Read the model definition and answer for the solid it produces. Units are mm, in the model's axes. A direction names the side the tool comes from. Coordinates: 2 decimals unless noted, no trailing zeros. Order: outer loops, then holes, each group sorted by start corner. A loop starts at its lowest first (then second) coordinate and runs counter-clockwise, first axis right, second up. Notation, with made-up numbers: M 65.25,-0.5 L 111.25,-0.5 A22 ccw 111.25,35.5 Z; hole C 58,40.5 d6. An arc over 180 degrees is marked long. Put each result on its own line as item: value.
from build123d import *

# Parameters (mm, degrees)
SKETCH1_R             = 2.25
SKETCH1_R_2           = 1.25
BOSS_EXTRUDE1_DEPTH   = 10
BOSS_EXTRUDE1_2_DEPTH = 10
BOSS_EXTRUDE1_3_DEPTH = 10
BOSS_EXTRUDE1_4_DEPTH = 10
SKETCH1_3_W           = 117
SKETCH1_3_H           = 35
BOSS_EXTRUDE2_DEPTH   = 2
SKETCH1_4_W           = 65
SKETCH1_4_H           = 35
BOSS_EXTRUDE3_DEPTH   = 10
FILLET1_R             = 2


with BuildPart() as part:
    # Sketch1 → Boss-Extrude1 (new body)
    with BuildSketch(Plane.XY):
        with Locations((-38.5, -11.5)):
            Circle(SKETCH1_R)
        with Locations((-38.5, -11.5)):
            Circle(SKETCH1_R_2, mode=Mode.SUBTRACT)
    extrude(amount=BOSS_EXTRUDE1_DEPTH)



with BuildPart() as body_2:
    # Sketch1 → Boss-Extrude1 2 (new body)
    with BuildSketch(Plane.XY):
        with Locations((-11.5, -11.5)):
            Circle(SKETCH1_R)
        with Locations((-11.5, -11.5)):
            Circle(SKETCH1_R_2, mode=Mode.SUBTRACT)
    extrude(amount=BOSS_EXTRUDE1_2_DEPTH)


with BuildPart() as body_3:
    # Sketch1 → Boss-Extrude1 3 (new body)
    with BuildSketch(Plane.XY):
        with Locations((-11.5, 11.5)):
            Circle(SKETCH1_R)
        with Locations((-11.5, 11.5)):
            Circle(SKETCH1_R_2, mode=Mode.SUBTRACT)
    extrude(amount=BOSS_EXTRUDE1_3_DEPTH)


with BuildPart() as body_4:
    # Sketch1 → Boss-Extrude1 4 (new body)
    with BuildSketch(Plane.XY):
        with Locations((-38.5, 11.5)):
            Circle(SKETCH1_R)
        with Locations((-38.5, 11.5)):
            Circle(SKETCH1_R_2, mode=Mode.SUBTRACT)
    extrude(amount=BOSS_EXTRUDE1_4_DEPTH)


with BuildPart() as part_1:
    add(part.part)

    add(body_2.part)  # Boss-Extrude2 merges body 2

    add(body_3.part)  # Boss-Extrude2 merges body 3

    add(body_4.part)  # Boss-Extrude2 merges body 4
    # Sketch1<3> → Boss-Extrude2 (add)
    with BuildSketch(Plane.XY):
        Rectangle(SKETCH1_3_W, SKETCH1_3_H)
    extrude(amount=BOSS_EXTRUDE2_DEPTH)

    # Sketch1<4> → Boss-Extrude3 (add)
    with BuildSketch(Plane.XY):
        with Locations((26, 0)):
            Rectangle(SKETCH1_4_W, SKETCH1_4_H)
    extrude(amount=BOSS_EXTRUDE3_DEPTH)

    # Fillet1
    fillet1_edges = [part_1.edges().sort_by_distance(p)[0] for p in [
        (-58.5, 17.5, 1),
        (58.5, 17.5, 5),
        (58.5, -17.5, 5),
        (-58.5, -17.5, 1),
        (-6.5, -17.5, 6),
        (-6.5, 17.5, 6),
    ]]
    fillet(fillet1_edges, radius=FILLET1_R)


solid = part_1.part
Q1. Find section B-B on y = -11.5. Write down the section's boundary in (x, z).
Answers below:
outline: M -58.5,0 L 58.5,0 L 58.5,10 L -6.5,10 L -6.5,2 L -9.25,2 L -9.25,10 L -10.25,10 L -10.25,2 L -12.75,2 L -12.75,10 L -13.75,10 L -13.75,2 L -36.25,2 L -36.25,10 L -37.25,10 L -37.25,2 L -39.75,2 L -39.75,10 L -40.75,10 L -40.75,2 L -58.5,2 Z
Q2. A tool of negligible diameter and unlimited length cuts with its end or side. For faces 4 (the face through (-12.421, -10.655, 5.944)), 5 (the face through (-5.9, -16.93, 6.06)), 6 (the face through (-10.5, 10.5, 10)), 7 (the face through (57.9, -16.93, 5.07)), 8 (the face through (-6.5, 0, 6)), from which of +Z, -Z, +X, -X, +Y, -Y can it reach the whole face along a straight path? Write none if from no direction.
Answers below:
face 4: +Z
face 5: +Z, -X, -Y
face 6: +Z, +X, -X, +Y, -Y
face 7: +Z, -Z, +X, -Y
face 8: +Z, +Y, -Y
Q3. Find section A-A on z = 7. Give the number of separate pieces and of enclosed holes in the cut face, plus the area to 3 significant figures.
Answers below:
separate pieces: 5
enclosed holes: 4
area: 2,320 mm^2
Q4. Find section D-D on y = 1. Write down the section's boundary in (x, z).
Answers below:
outline: M -58.5,0 L 58.5,0 L 58.5,10 L -6.5,10 L -6.5,2 L -58.5,2 Z
Q5. Find section C-C on x = -11.5. Write down the section's boundary in (y, z).
Answers below:
outline: M -17.5,0 L 17.5,0 L 17.5,2 L 13.75,2 L 13.75,10 L 12.75,10 L 12.75,2 L 10.25,2 L 10.25,10 L 9.25,10 L 9.25,2 L -9.25,2 L -9.25,10 L -10.25,10 L -10.25,2 L -12.75,2 L -12.75,10 L -13.75,10 L -13.75,2 L -17.5,2 Z
Q6. Given pin 1 (1.5 mm diameter, centred on x = -11.5, y = 11.5, fed in from +Z), flat-ended and moving along its own axis, determine where the tip first touches the part or whether it passes through.
Answers below:
pin 1: stops at z = 2
Q7. Consider line 1 along Y through (x, z) = (-11.5, 5); line 2 along X through (y, z) = (-11.5, 6.25); line 3 along X through (y, z) = (-2.5, 2.25). Determine where each line is inside the solid, lowest interval first.
Answers below:
line 1: y = -13.75 to -12.75, -10.25 to -9.25, 9.25 to 10.25, 12.75 to 13.75
line 2: x = -40.75 to -39.75, -37.25 to -36.25, -13.75 to -12.75, -10.25 to -9.25, -6.5 to 58.5
line 3: x = -6.5 to 58.5
Q8. For a pull along Y with two mould halves and no side action, classify faces 1 (the face through (12, 17.5, 4)), 2 (the face through (-39.421, 12.345, 5.944)), 3 (the face through (-10.5, -12.5, 10)) as +Y half, -Y half, draft (parallel to the pull), parting line (faces both ways), or undercut.
Answers below:
face 1: +Y half
face 2: undercut
face 3: draft
